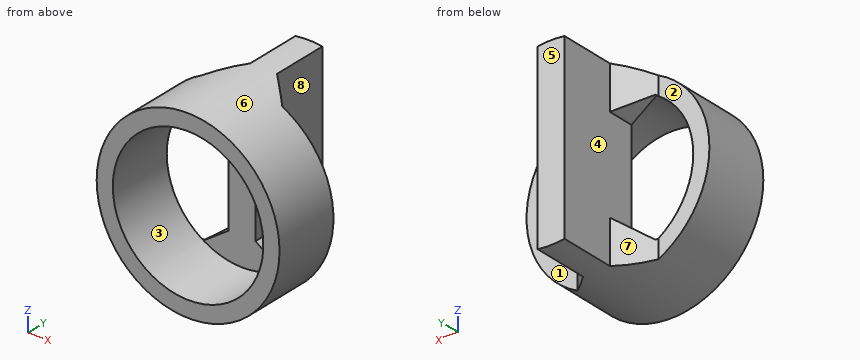
Autodesk Inventor part; units mm, degrees
ref_plane "YZ Plane" through (0, 0, 0) normal (1, 0, 0) x (0, 1, 0)
ref_plane "XZ Plane" through (0, 0, 0) normal (0, 1, 0) x (-1, 0, 0)
ref_plane "XY Plane" through (0, 0, 0) normal (0, 0, 1) x (1, 0, 0)
sketch "스케치1" plane through (0, 0, 0) normal (0, 1, 0) x (-1, 0, 0)
  circle A0 centre (0, 0) radius 2.8
  circle A1 centre (0, 0) radius 3.4
  dimension "d0" = 5.6
  dimension "d1" = 6.8
extrude "돌출1" add sketch "스케치1" along normal blind 2.5
sketch "스케치2" plane through (0, 2.5, 0) normal (0, 1, 0) x (1, 0, 0)
  circle A0 centre (0, 0) radius 3.4
  circle A1 centre (0, 0) radius 3.4
  line L0 (0.5, 3.363) -> (-0.5, 3.363)
  line L1 (-0.5, 3.363) -> (-0.5, -3.363)
  line L2 (-0.5, -3.363) -> (0.5, -3.363)
  line L3 (0.5, -3.363) -> (0.5, 3.363)
  line L4 (0.5, 3.363) -> (-0.5, -3.363) construction
  line L5 (-0.5, 3.363) -> (0.5, -3.363) construction
  point P0 (-0.5, -3.363)
  point P1 (0.5, -3.363)
  point P2 (0.5, 3.363)
  point P3 (-0.5, 3.363)
  dimension "d4" = 1
extrude "돌출2" add sketch "스케치2" along normal blind 3.1 contours L0 A0 | L3 L2 L1 L0 | A0 L2
chamfer "모따기1" distance 1 angle 45 4 edges at (0.5, 2.5, 3.059) (0.5, 2.5, -3.059) (-0.5, 2.5, -3.059) (-0.5, 2.5, 3.059)
chamfer "모따기2" distance 1 angle 45 4 edges at (-0.5, 3, -2.755) (-0.5, 3, 2.755) (0.5, 3, 2.755) (0.5, 3, -2.755)
properties part number "terminalcap_4.1mm_addon_large"
Check sheet for the modelled part. Datum: model origin and axes. Units: mm. Face numbers are marked on the shaded views. A direction names the side the tool comes from. Round coordinates to 2 decimals unless told otherwise and drop trailing zeros. Loops run counter-clockwise (first coordinate to the right, second up) from the corner with the lowest first, then second, coordinate; pieces in that order, holes last. Notation, with made-up numbers: M 29,13 L 66,13 A17 ccw 66,45 Z; hole C 34.5,-30 d9. An arc over 180 degrees is marked long. Answer as a JSON object with one key per item and string values.
1. Scan lines: line 1 (X direction, y = 1.9, z = 0); line 2 (X direction, y = 2.9, z = 0.25). Record each from-to range of solid material in increasing order.
Reply:
{"line 1": "x = -3.4 to -2.8, 2.8 to 3.4", "line 2": "x = -0.5 to 0.5"}
2. Mould release check, pull along Z, two halves, no side actions. Record for the marked faces 6, 7 and 8: pulls with the +Z half, pulls with the -Z half, needs draft (parallel to the pull), parting line crosses it, or undercut.
Reply:
{"face 6": "parting line crosses it", "face 7": "needs draft", "face 8": "undercut"}
3. Access from +Z, -Z, +X, -X, +Y, -Y to the whole of each face (thin tool, end or side, straight path). Record for the marked faces 1, 2, 3, 4 and 5.
Reply:
{"face 1": "+Z, -Z, +X, +Y", "face 2": "+Z, -Z, -X, +Y", "face 3": "-Y", "face 4": "-X, +Y", "face 5": "+Z, -Z, +X, -X, +Y"}
4. Section check A-A (z = 0). Record the boundary of the cut face in (x, y).
Reply:
{"outline": "M -3.4,0 L -2.8,0 L -2.8,2.5 L -3.4,2.5 Z; M -0.5,2.5 L 0.5,2.5 L 0.5,5.6 L -0.5,5.6 Z; M 2.8,0 L 3.4,0 L 3.4,2.5 L 2.8,2.5 Z"}
5. Section check C-C (x = 0.75). Record the boundary of the cut face in (y, z).
Reply:
{"outline": "M 0,-3.32 L 3.25,-3.32 L 3.25,-1.93 L 2.5,-1.93 L 2.5,-2.7 L 0,-2.7 Z; M 0,2.7 L 2.5,2.7 L 2.5,1.93 L 3.25,1.93 L 3.25,3.32 L 0,3.32 Z"}
6. Section check D-D (y = 1.7). Record the boundary of the cut face in (x, z).
Reply:
{"outline": "C 0,0 d6.8; hole C 0,0 d5.6"}
7. Section check B-B (x = 0). Record the boundary of the cut face in (y, z).
Reply:
{"outline": "M 0,-3.4 L 5.6,-3.4 L 5.6,3.4 L 0,3.4 L 0,2.8 L 2.5,2.8 L 2.5,-2.8 L 0,-2.8 Z"}
8. Gauge pin test, flat ends, axial feed: P1, Ø2, axis at x = -3, z = 0.5, coming from the +Y side; P2, Ø1.5, axis at y = 1, z = 1, coming from the +X side; P3, Ø0.9, axis at x = 0, z = -0.5, coming from the -Y side. Record the tip position at first contact, or that the pin passes through.
Reply:
{"P1": "stops at y = 2.5", "P2": "stops at x = 3.39", "P3": "stops at y = 2.5"}
